The figure shows three views and two pictorial views of one solid part (mm, origin at its lowest corner). Answer the questions. A direction names the side the tool comes from. Round coordinates to 2 decimals unless told otherwise and drop trailing zeros. Write each loop counter-clockwise with the first axis right and the second up, starting at its lowest first coordinate (ties: lowest second). Pieces come first, ordered by that corner, then holes. Notation, with made-up numbers: M -34.5,-35.75 L -26.5,-35.75 A25 cw -26.5,-19.75 Z; hole C -9,89.5 d10. An arc over 180 degrees is marked long. Answer in a Markdown table with one row per item.
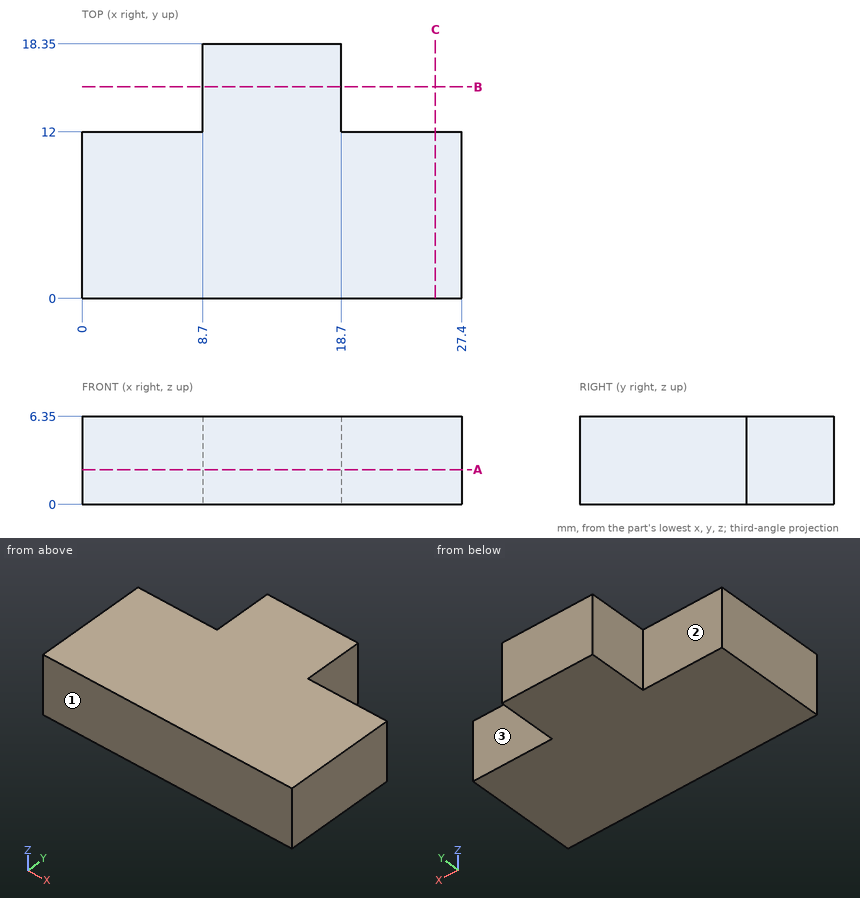
1. The part is cut by section C-C (x = 25.5). Determine the outline of the cut face in (y, z).
Calculated:
| item | result |
|---|---|
| outline | M 0,0 L 12,0 L 12,6.35 L 0,6.35 Z |
2. Consider line 1 along Y through (x, z) = (19.25, 5.25); line 2 along X through (y, z) = (15, 5.25). Determine where each line is inside the solid, lowest interval first. Write a range as from..to.
Calculated:
| item | result |
|---|---|
| line 1 | y = 0..12 |
| line 2 | x = 8.7..18.7 |
3. A tool of negligible diameter and unlimited length cuts with its end or side. For the marked faces 1, 2 and 3, from which of +Z, -Z, +X, -X, +Y, -Y can it reach the whole face along a straight path? Write none if from no direction.
Calculated:
| item | result |
|---|---|
| face 1 | +Z, -Z, +X, -X, -Y |
| face 2 | +Z, -Z, -X, +Y |
| face 3 | +Z, -Z, +X, +Y |
4. Given pin 1 (3 mm diameter, centred on x = 23.5, y = 15, fed in from +Z); pin 2 (3 mm diameter, centred on x = 22, z = 4, fed in from +Y), each flat-ended and moving along its own axis, determine where each tip first touches the part or whether it passes through.
Calculated:
| item | result |
|---|---|
| pin 1 | passes through |
| pin 2 | stops at y = 12 |
5. The part is cut by section A-A (z = 2.5). Determine the outline of the cut face in (x, y), plus the area to 3 significant figures.
Calculated:
| item | result |
|---|---|
| outline | M 0,0 L 27.4,0 L 27.4,12 L 18.7,12 L 18.7,18.35 L 8.7,18.35 L 8.7,12 L 0,12 Z |
| area | 392 mm² |
6. The part is cut by section B-B (y = 15.25). Determine the outline of the cut face in (x, z).
Calculated:
| item | result |
|---|---|
| outline | M 8.7,0 L 18.7,0 L 18.7,6.35 L 8.7,6.35 Z |
